Model file for the job. Use its own axes, mm. Face numbers are marked on the shaded views. A direction names the side the tool comes from. Coordinates: 2 decimals unless noted, no trailing zeros. Loops run counter-clockwise (first coordinate to the right, second up) from the corner with the lowest first, then second, coordinate; pieces in that order, holes last. Notation, with made-up numbers: M 0,37.5 L 34,37.5 A24 cw 34,53.5 Z; hole C 84.25,8 d8. An arc over 180 degrees is marked long. Write item = value, one per line. Start each with the question number.
from build123d import *

# Parameters (mm, degrees)
F0_R     = 4
F1_DEPTH = 3
F2_R     = 2.5
F3_DEPTH = 30
F4_R     = 4
F4_R_2   = 2.5
F5_DEPTH = 3


with BuildPart() as f1:
    # F0 (on Front) → F1 (new body)
    with BuildSketch(Plane.XZ):
        Circle(F0_R)
    extrude(amount=F1_DEPTH)

    # F2 (on face) → F3 (join)
    with BuildSketch(Plane.XZ.offset(3)):
        Circle(F2_R)
    extrude(amount=F3_DEPTH)

    # F4 (on face) → F5 (join)
    with BuildSketch(Plane.XZ.offset(33)):
        Circle(F4_R)
        Circle(F4_R_2, mode=Mode.SUBTRACT)
        Circle(F4_R_2)
    extrude(amount=F5_DEPTH)


solid = f1.part
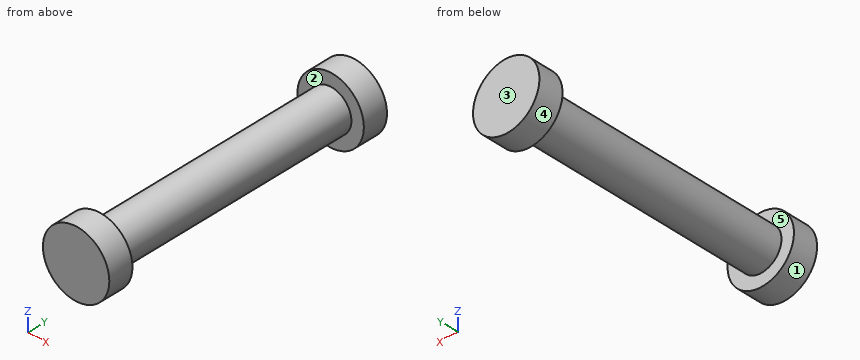
Item 1: Probe L1, parallel to Y at x = -0.5, z = -3; L2, parallel to Z at x = 0, y = -23; L3, parallel to Z at x = 0.5, y = -22. List the from-to ranges inside material, lowest first.
Item 2: Pin check, flat tips, straight feed: pin 1 Ø2 at (y, z) = (-12.5, 0.5) entering from +X; pin 2 Ø1 at (x, y) = (-2.5, -16.5) entering from -Z; pin 3 Ø1.5 at (y, z) = (-9, -1.5) entering from +X. Stop position of each tip, or through.
Item 3: Cut at C-C (x = 0). Give the cut face in (y, z), plus the area to 3 significant figures.
Item 4: Pull direction Y, two halves, no side cores. Call the marked faces 1, 2 and 3: +Y half, -Y half, draft (parallel to the pull), parting line (faces both ways), or undercut.
Item 5: Cut at D-D (z = -3.25). Give the cut face in (x, y).
Item 6: Cut at A-A (x = 3.25). Give the cut face in (y, z), plus the area to 3 significant figures.
Item 7: Cut at B-B (z = 0). Give the cut face in (x, y).
Item 8: 3-axis set-ups, long thin cutter, end or side, ignore diameter. For the marked faces 4 and 5: which of +Z, -Z, +X, -X, +Y, -Y reach the whole face in a straight line?
Reported:
q1.L1 = -36 to -33, -3 to 0
q1.L2 = -2.5 to 2.5
q1.L3 = -2.45 to 2.45
q2.pin_1 = 2.5
q2.pin_2 = -1.5
q2.pin_3 = 2.38
q3.outline = M -36,-4 L -33,-4 L -33,-2.5 L -3,-2.5 L -3,-4 L 0,-4 L 0,4 L -3,4 L -3,2.5 L -33,2.5 L -33,4 L -36,4 Z
q3.area = 198 mm^2
q4.face_1 = draft
q4.face_2 = undercut
q4.face_3 = +Y half
q5.outline = M -2.33,-36 L 2.33,-36 L 2.33,-33 L -2.33,-33 Z; M -2.33,-3 L 2.33,-3 L 2.33,0 L -2.33,0 Z
q6.outline = M -36,-2.33 L -33,-2.33 L -33,2.33 L -36,2.33 Z; M -3,-2.33 L 0,-2.33 L 0,2.33 L -3,2.33 Z
q6.area = 28.0 mm^2
q7.outline = M -4,-36 L 4,-36 L 4,-33 L 2.5,-33 L 2.5,-3 L 4,-3 L 4,0 L -4,0 L -4,-3 L -2.5,-3 L -2.5,-33 L -4,-33 Z
q8.face_4 = +Y, -Y
q8.face_5 = none
